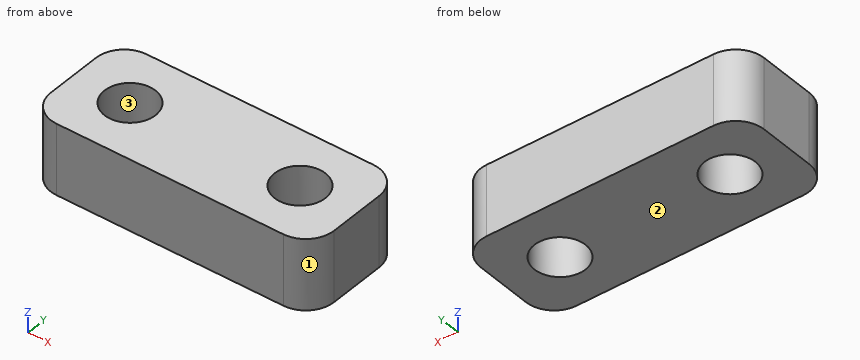
```python
from build123d import *

# Parameters (mm, degrees)
SKETCH2_W            = 20
SKETCH2_H            = 8
BOSS_EXTRUDE1_DEPTH  = 5
M3_CLEARANCE_HOLE1_D = 3.6
FILLET1_R            = 2


with BuildPart() as part:
    # Sketch2 → Boss-Extrude1 (new body)
    with BuildSketch(Plane.XY):
        with Locations((10, 4)):
            Rectangle(SKETCH2_W, SKETCH2_H)
    extrude(amount=BOSS_EXTRUDE1_DEPTH)

    # M3 Clearance Hole1 (through all)
    with Locations(Plane.XY.offset(5)):
        with Locations((4, 4), (16, 4)):
            Hole(M3_CLEARANCE_HOLE1_D / 2)

    # Fillet1
    fillet1_edges = [part.edges().sort_by_distance(p)[0] for p in [
        (0, 8, 2.5),
        (20, 8, 2.5),
        (20, 0, 2.5),
        (0, 0, 2.5),
    ]]
    fillet(fillet1_edges, radius=FILLET1_R)


solid = part.part
```
Build history of the part. All positions in model axes, mm. Face numbers are marked on the shaded views. Round coordinates to 2 decimals unless told otherwise and drop trailing zeros. Write each loop counter-clockwise with the first axis right and the second up, starting at its lowest first coordinate (ties: lowest second). Pieces come first, ordered by that corner, then holes.
1) Band-saw the part on B-B, the plane x = 4. List the corners of the cut face in (y, z).
2) Band-saw the part on C-C, the plane z = 3.25. List the corners of the cut face in (x, y), and give its area (3 significant figures).
3) Mould opens along Y. For the marked faces 1, 2 and 3 say: +Y half, -Y half, draft (parallel to the pull), parting line (faces both ways), or undercut.
4) Band-saw the part on A-A, the plane y = 4. List the corners of the cut face in (x, z), and give its area (3 significant figures).
5) Drill centre lines: probe 1 along X at (y, z) = (5.5, 0.35); probe 2 along Y at (x, z) = (4, 3.55); probe 3 along X at (y, z) = (3.25, 4.55). Where is each one in solid material? Low to high.
6) Pin check, flat tips, straight feed: pin 1 (3 mm diameter, centred on x = 4, y = 4, fed in from +Z); pin 2 (1.5 mm diameter, centred on y = 1, z = 2, fed in from -X). Stop position of each tip, or through.
7) Band-saw the part on D-D, the plane x = 15. List the corners of the cut face in (y, z), and give its area (3 significant figures).
Ans:
1. outline: (0, 0) - (2.2, 0) - (2.2, 5) - (0, 5) - close; (5.8, 0) - (8, 0) - (8, 5) - (5.8, 5) - close
2. outline: (0, 2) arc R2 ccw to (2, 0) - (18, 0) arc R2 ccw to (20, 2) - (20, 6) arc R2 ccw to (18, 8) - (2, 8) arc R2 ccw to (0, 6) - close; hole circle Ø3.6 at (4, 4); hole circle Ø3.6 at (16, 4)
2. area: 136 mm2
3. face 1: -Y half
3. face 2: draft
3. face 3: undercut
4. outline: (0, 0) - (2.2, 0) - (2.2, 5) - (0, 5) - close; (5.8, 0) - (14.2, 0) - (14.2, 5) - (5.8, 5) - close; (17.8, 0) - (20, 0) - (20, 5) - (17.8, 5) - close
4. area: 64.0 mm2
5. probe 1: x = 0 to 3.01, 4.99 to 15.01, 16.99 to 20
5. probe 2: y = 0 to 2.2, 5.8 to 8
5. probe 3: x = 0 to 2.36, 5.64 to 14.36, 17.64 to 20
6. pin 1: passes through
6. pin 2: stops at x = 0.02
7. outline: (0, 0) - (2.5, 0) - (2.5, 5) - (0, 5) - close; (5.5, 0) - (8, 0) - (8, 5) - (5.5, 5) - close
7. area: 25.0 mm2
